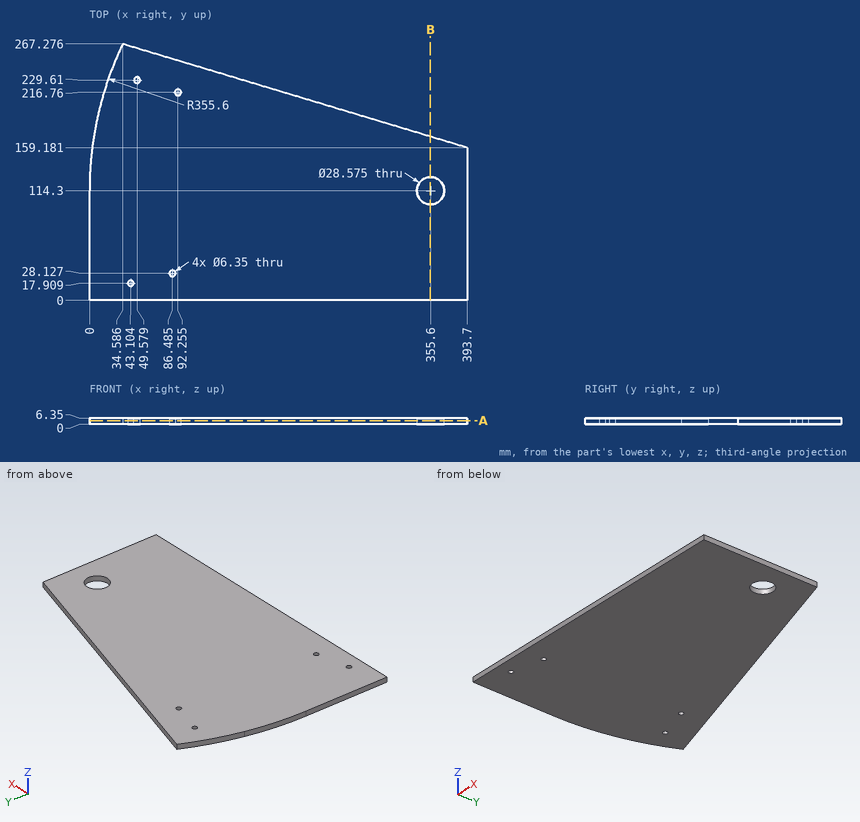
Here's the drawing with two shaded views (mm, measured from the low corner). I have some questions. Give positions to 0.01 mm unless a question says otherwise; leave off trailing zeros. Loops run counter-clockwise (first coordinate to the right, second up) from the corner with the lowest first, then second, coordinate; pieces in that order, holes last. Notation, with made-up numbers: (89, 71) -> (120, 71) arc R15 cw to (120, 79) -> close; hole circle Ø9 at (-28.75, 58.25). An arc over 180 degrees is marked (long way). Use one line per item in the form item = value.
1) Will this pin go through, and if not, where does the flat tip stop? pin 1 (3 mm diameter, centred on x = 125.5, z = 4, fed in from +Y).
Answers:
pin_1 = 240.36
2) I need wall thicknesses on line 1 along Y through (x, z) = (355.6, 4); line 2 along Y through (x, z) = (124.5, 3.75); line 3 along Y through (x, z) = (105.5, 3.25). Which ranges of each line are inside material? Lowest first, please.
Answers:
line_1 = 0 to 100.01, 128.59 to 170.65
line_2 = 0 to 240.21
line_3 = 0 to 245.93
3) If we section it at A-A (z = 4): Count the separate pieces of the cut face and the enclosed holes in it, plus the area to 3 significant figures.
Answers:
separate_pieces = 1
enclosed_holes = 5
area = 83,300 mm²
4) If we section it at B-B (x = 355.5): Please give me the cut outline in (y, z).
Answers:
outline = (0, 0) -> (100.01, 0) -> (100.01, 6.35) -> (0, 6.35) -> close; (128.59, 0) -> (170.68, 0) -> (170.68, 6.35) -> (128.59, 6.35) -> close
